Geometry: final body of the model. Coordinates: model frame, mm. Round coordinates to 2 decimals unless told otherwise and drop trailing zeros. Loops run counter-clockwise (first coordinate to the right, second up) from the corner with the lowest first, then second, coordinate; pieces in that order, holes last. Notation, with made-up numbers: M 51.5,28.25 L 100.5,28.25 A18 ccw 100.5,45.25 Z; hole C 67.25,37 d5. An arc over 180 degrees is marked long. Answer as a JSON object with one key per item and string values.
from build123d import *

# Parameters (mm, degrees)
SKETCH1_W           = 120
SKETCH1_H           = 83
BOSS_EXTRUDE1_DEPTH = 13
SKETCH2_W           = 6
SKETCH2_H           = 50
CUT_EXTRUDE1_DEPTH  = 6
SKETCH4_W           = 1.557692307
SKETCH4_H           = 0.75
BOSS_EXTRUDE3_DEPTH = 3
SKETCH5_W           = 3.5
SKETCH5_H           = 5
BOSS_EXTRUDE4_DEPTH = 1


with BuildPart() as part:
    # Sketch1 → Boss-Extrude1 (new body)
    with BuildSketch(Plane.XY):
        Rectangle(SKETCH1_W, SKETCH1_H)
    extrude(amount=BOSS_EXTRUDE1_DEPTH)

    # Sketch2 → Cut-Extrude1 (cut)
    with BuildSketch(Plane.XY.offset(13)):
        with Locations((-42.602242675, 7.231357776)):
            Rectangle(SKETCH2_W, SKETCH2_H)
        with Locations((0.647757325, 7.231357776)):
            Rectangle(SKETCH2_W, SKETCH2_H)
        with Locations((43.897757325, 7.231357776)):
            Rectangle(SKETCH2_W, SKETCH2_H)
    extrude(amount=-CUT_EXTRUDE1_DEPTH, mode=Mode.SUBTRACT)

    # Sketch4 → Boss-Extrude3 (add)
    # profile 1 of 6: a face of its own
    with BuildSketch(Plane.XY.offset(13)):
        Polygon((28.787603371, -32.130057538), (29.621437506, -32.130057538), (30.287603371, -35.002954173), (31.051125006, -32.130057538), (31.834478371, -32.130057538), (32.595295679, -35.002954173), (33.257855775, -32.130057538), (34.095295679, -32.130057538), (33.055031256, -36.630057538), (32.211281256, -36.630057538), (31.441449525, -33.721103211), (30.668012025, -36.630057538), (29.830572121, -36.630057538), align=None)
    # profile 2 of 6: a face of its own
    with BuildSketch(Plane.XY.offset(13)):
        Polygon((37.930932698, -32.130057538), (38.68183414, -32.130057538), (40.499141833, -36.630057538), (39.636461544, -36.630057538), (39.286701929, -35.706980615), (37.327867794, -35.706980615), (36.977206736, -36.630057538), (36.114526448, -36.630057538), align=None)
        Polygon((38.30683414, -33.337088788), (37.634358179, -34.899288307), (38.980211544, -34.899288307), align=None, mode=Mode.SUBTRACT)
    # profile 3 of 6: a face of its own
    with BuildSketch(Plane.XY.offset(13)):
        Polygon((42.893372602, -32.130057538), (43.701064909, -32.130057538), (43.701064909, -35.82236523), (44.970295679, -35.82236523), (44.970295679, -36.630057538), (42.893372602, -36.630057538), align=None)
    # profile 4 of 6: a face of its own
    with BuildSketch(Plane.XY.offset(13)):
        Polygon((47.393372602, -32.130057538), (48.201064909, -32.130057538), (48.201064909, -35.82236523), (49.470295679, -35.82236523), (49.470295679, -36.630057538), (47.393372602, -36.630057538), align=None)
    # profile 5 of 6: a face of its own
    with BuildSketch(Plane.XY.offset(13)):
        with Locations((52.672218756, -34.985826769)):
            Rectangle(SKETCH4_W, SKETCH4_H)
    # profile 6 of 6: a face of its own
    with BuildSketch(Plane.XY.offset(13)):
        Polygon((56.220295679, -32.130057538), (58.643372602, -32.130057538), (58.643372602, -32.937749846), (57.027987986, -32.937749846), (57.027987986, -33.803134461), (58.643372602, -33.803134461), (58.643372602, -34.610826769), (57.027987986, -34.610826769), (57.027987986, -35.82236523), (58.643372602, -35.82236523), (58.643372602, -36.630057538), (56.220295679, -36.630057538), align=None)
    extrude(amount=BOSS_EXTRUDE3_DEPTH)

    # Sketch5 → Boss-Extrude4 (add)
    with BuildSketch(Plane.XY.offset(13)):
        with Locations((57.43183414, -34.380057538)):
            Rectangle(SKETCH5_W, SKETCH5_H)
    extrude(amount=BOSS_EXTRUDE4_DEPTH)


solid = part.part
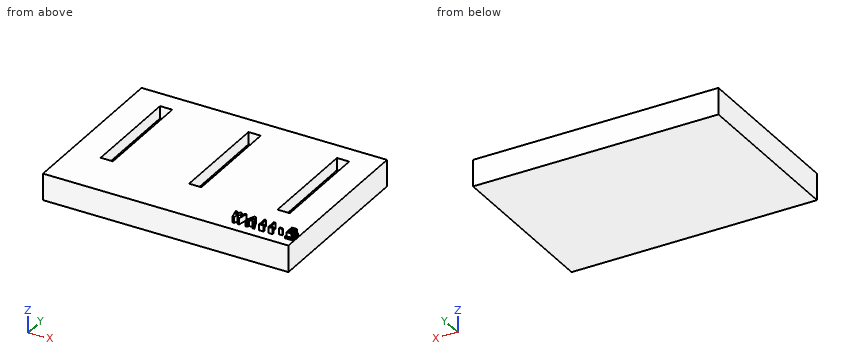
1) Pin query (flat end, axial travel): P1, Ø0.5, axis at x = 52.5, z = 14.5, coming from the +Y side; P2, Ø1.3, axis at x = 58, z = 15, coming from the +Y side; P3, Ø0.6, axis at y = -35, z = 14, coming from the +X side; P4, Ø10, axis at x = -38, y = 21.5, coming from the -Z side. Return the tip coordinate at first contact, or that it passes through.
Results:
{"P1": "y = -34.61", "P2": "y = -32.13", "P3": "x = 59.18", "P4": "z = 0"}
2) Ray query, line 1 (X direction, y = -14.5, z = 8.5); line 2 (Y direction, x = -1.5, z = 7.5); line 3 (Z direction, x = 53, y = -13.5). Return the intervals inside material, ascending.
Results:
{"line 1": "-60 to -45.6, -39.6 to -2.35, 3.65 to 40.9, 46.9 to 60", "line 2": "-41.5 to -17.77, 32.23 to 41.5", "line 3": "0 to 13"}
3) Section query C-C (x = -32.5). Return the cut outline in (y, z), and give its area (3 significant figures).
Results:
{"outline": "M -41.5,0 L 41.5,0 L 41.5,13 L -41.5,13 Z", "area": "1,080 mm2"}
4) Section query D-D (y = -28.5). Return the cut outline in (x, z), and give its area (3 significant figures).
Results:
{"outline": "M -60,0 L 60,0 L 60,13 L -60,13 Z", "area": "1,560 mm2"}
5) Section query B-B (y = -4). Return the cut outline in (x, z).
Results:
{"outline": "M -60,0 L 60,0 L 60,13 L 46.9,13 L 46.9,7 L 40.9,7 L 40.9,13 L 3.65,13 L 3.65,7 L -2.35,7 L -2.35,13 L -39.6,13 L -39.6,7 L -45.6,7 L -45.6,13 L -60,13 Z"}
6) Section query A-A (z = 9.5). Return the cut outline in (x, y).
Results:
{"outline": "M -60,-41.5 L 60,-41.5 L 60,41.5 L -60,41.5 Z; hole M -45.6,-17.77 L -39.6,-17.77 L -39.6,32.23 L -45.6,32.23 Z; hole M -2.35,-17.77 L 3.65,-17.77 L 3.65,32.23 L -2.35,32.23 Z; hole M 40.9,-17.77 L 46.9,-17.77 L 46.9,32.23 L 40.9,32.23 Z"}
